CAD build for the part. Positions are in the model's coordinates, mm. A direction names the side the tool comes from. Give positions to 0.01 mm unless a question says otherwise; leave off trailing zeros. Loops run counter-clockwise (first coordinate to the right, second up) from the corner with the lowest first, then second, coordinate; pieces in that order, holes last. Notation, with made-up numbers: M 83,39 L 135,39 A15 cw 135,45 Z; hole C 9.5,-3.75 d8. An arc over 180 degrees is marked long. One line per question, with ' | ' between items.
Autodesk Inventor part; units mm, degrees
ref_plane "YZ Plane" through (0, 0, 0) normal (1, 0, 0) x (0, 1, 0)
ref_plane "XZ Plane" through (0, 0, 0) normal (0, 1, 0) x (-1, 0, 0)
ref_plane "XY Plane" through (0, 0, 0) normal (0, 0, 1) x (1, 0, 0)
sketch "Sketch1" plane through (0, 0, 0) normal (1, 0, 0) x (0, 1, 0)
  line L0 (0, 0) -> (0, -127)
  line L1 (0, -127) -> (10, -127)
  line L2 (10, -127) -> (10, -101.6)
  line L3 (10, -101.6) -> (20, -101.6)
  line L4 (20, -101.6) -> (20, 0)
  line L5 (20, 0) -> (0, 0)
  dimension "d0" = 127
  dimension "d1" = 10
  dimension "d2" = 25.4
  dimension "d3" = 10
extrude "Extrusion1" add sketch "Sketch1" along normal blind 863.6
chamfer "Chamfer1" distance 127 angle 45 1 edges at (863.6, 5, -127)
chamfer "Chamfer2" distance 127 angle 45 1 edges at (0, 5, -127)
properties part number "SkirtWidth" material "Wood (Birch)"
Item 1: Saw through at D-D on z = -64. Give the cut face in (x, y), and give its area (3 significant figures).
Conclusion:
outline: M 64,0 L 799.6,0 L 799.6,20 L 64,20 Z | area: 14,700 mm²
Item 2: Drop flat-ended pins along their axis: P1, Ø8, axis at x = 539, y = 16, coming from the -Z side; P2, Ø2, axis at y = 13.5, z = -59.5, coming from the -X side; P3, Ø20.5, axis at x = 510.5, z = -116.5, coming from the +Y side. Give the stop position or say it passes through.
Conclusion:
P1: z = -101.6 | P2: x = 58.5 | P3: y = 10
Item 3: 3-axis set-ups, long thin cutter, end or side, ignore diameter. For faces 1 (the flat face through (426, 0, -63)), 2 (the flat face through (427, 10, -114)): which of +Z, -Z, +X, -X, +Y, -Y reach the whole face in a straight line?
Conclusion:
face 1: +Z, -Z, +X, -X, -Y | face 2: -Z, +X, -X, +Y
Item 4: Saw through at B-B on x = 679. Give the cut face in (y, z).
Conclusion:
outline: M 0,-127 L 10,-127 L 10,-101.6 L 20,-101.6 L 20,0 L 0,0 Z
Item 5: Drill centre lines: line 1 along Z through (x, y) = (513, 15); line 2 along Y through (x, z) = (364, -111.5); line 3 along X through (y, z) = (12, -40.5). Where is each one in solid material? Low to high. Write a range as [from, to].
Conclusion:
line 1: [-101.6, 0] | line 2: [0, 10] | line 3: [40.5, 823.1]
Item 6: Saw through at C-C on z = -32. Give the cut face in (x, y), and give its area (3 significant figures).
Conclusion:
outline: M 32,0 L 831.6,0 L 831.6,20 L 32,20 Z | area: 16,000 mm²
